from build123d import *

# Parameters (mm, degrees)
F0_W          = 19
F0_H          = 16
F1_DEPTH      = 200
F1_DEPTH_BACK = 25
F3_DEPTH      = 8


with BuildPart() as f1:
    # F0 (on Top) → F1 (new body, two sides)
    with BuildSketch(Plane.XY) as f1_sk:
        with Locations((4.5, 0)):
            Rectangle(F0_W, F0_H)
    extrude(amount=F1_DEPTH)
    extrude(f1_sk.sketch, amount=-F1_DEPTH_BACK)

    # F2 (on Front) → F3 (join, symmetric)
    with BuildSketch(Plane.XZ):
        with BuildLine():
            Line((-7.933333, 193.6), (-5, 191.4))
            Line((-5, 191.4), (-5, 197.4))
            Line((-5, 197.4), (-7.933333, 195.2))
            ThreePointArc((-7.933333, 195.2), (-8.333333, 194.4), (-7.933333, 193.6))
        make_face()
        with BuildLine():
            Line((-7.933333, 185.5), (-5, 183.3))
            Line((-5, 183.3), (-5, 189.3))
            Line((-5, 189.3), (-7.933333, 187.1))
            ThreePointArc((-7.933333, 187.1), (-8.333333, 186.3), (-7.933333, 185.5))
        make_face()
        with BuildLine():
            Line((-7.933333, 177.4), (-5, 175.2))
            Line((-5, 175.2), (-5, 181.2))
            Line((-5, 181.2), (-7.933333, 179))
            ThreePointArc((-7.933333, 179), (-8.333333, 178.2), (-7.933333, 177.4))
        make_face()
        with BuildLine():
            Line((-7.933333, 169.3), (-5, 167.1))
            Line((-5, 167.1), (-5, 173.1))
            Line((-5, 173.1), (-7.933333, 170.9))
            ThreePointArc((-7.933333, 170.9), (-8.333333, 170.1), (-7.933333, 169.3))
        make_face()
        with BuildLine():
            Line((-7.933333, 161.2), (-5, 159))
            Line((-5, 159), (-5, 165))
            Line((-5, 165), (-7.933333, 162.8))
            ThreePointArc((-7.933333, 162.8), (-8.333333, 162), (-7.933333, 161.2))
        make_face()
        with BuildLine():
            Line((-7.933333, 153.1), (-5, 150.9))
            Line((-5, 150.9), (-5, 156.9))
            Line((-5, 156.9), (-7.933333, 154.7))
            ThreePointArc((-7.933333, 154.7), (-8.333333, 153.9), (-7.933333, 153.1))
        make_face()
        with BuildLine():
            Line((-7.933333, 145), (-5, 142.8))
            Line((-5, 142.8), (-5, 148.8))
            Line((-5, 148.8), (-7.933333, 146.6))
            ThreePointArc((-7.933333, 146.6), (-8.333333, 145.8), (-7.933333, 145))
        make_face()
        with BuildLine():
            Line((-7.933333, 136.9), (-5, 134.7))
            Line((-5, 134.7), (-5, 140.7))
            Line((-5, 140.7), (-7.933333, 138.5))
            ThreePointArc((-7.933333, 138.5), (-8.333333, 137.7), (-7.933333, 136.9))
        make_face()
        with BuildLine():
            Line((-7.933333, 128.8), (-5, 126.6))
            Line((-5, 126.6), (-5, 132.6))
            Line((-5, 132.6), (-7.933333, 130.4))
            ThreePointArc((-7.933333, 130.4), (-8.333333, 129.6), (-7.933333, 128.8))
        make_face()
        with BuildLine():
            Line((-7.933333, 120.7), (-5, 118.5))
            Line((-5, 118.5), (-5, 124.5))
            Line((-5, 124.5), (-7.933333, 122.3))
            ThreePointArc((-7.933333, 122.3), (-8.333333, 121.5), (-7.933333, 120.7))
        make_face()
        with BuildLine():
            Line((-7.933333, 112.6), (-5, 110.4))
            Line((-5, 110.4), (-5, 116.4))
            Line((-5, 116.4), (-7.933333, 114.2))
            ThreePointArc((-7.933333, 114.2), (-8.333333, 113.4), (-7.933333, 112.6))
        make_face()
        with BuildLine():
            Line((-7.933333, 104.5), (-5, 102.3))
            Line((-5, 102.3), (-5, 108.3))
            Line((-5, 108.3), (-7.933333, 106.1))
            ThreePointArc((-7.933333, 106.1), (-8.333333, 105.3), (-7.933333, 104.5))
        make_face()
        with BuildLine():
            Line((-7.933333, 96.4), (-5, 94.2))
            Line((-5, 94.2), (-5, 100.2))
            Line((-5, 100.2), (-7.933333, 98))
            ThreePointArc((-7.933333, 98), (-8.333333, 97.2), (-7.933333, 96.4))
        make_face()
        with BuildLine():
            Line((-7.933333, 88.3), (-5, 86.1))
            Line((-5, 86.1), (-5, 92.1))
            Line((-5, 92.1), (-7.933333, 89.9))
            ThreePointArc((-7.933333, 89.9), (-8.333333, 89.1), (-7.933333, 88.3))
        make_face()
        with BuildLine():
            Line((-7.933333, 80.2), (-5, 78))
            Line((-5, 78), (-5, 84))
            Line((-5, 84), (-7.933333, 81.8))
            ThreePointArc((-7.933333, 81.8), (-8.333333, 81), (-7.933333, 80.2))
        make_face()
        with BuildLine():
            Line((-7.933333, 72.1), (-5, 69.9))
            Line((-5, 69.9), (-5, 75.9))
            Line((-5, 75.9), (-7.933333, 73.7))
            ThreePointArc((-7.933333, 73.7), (-8.333333, 72.9), (-7.933333, 72.1))
        make_face()
        with BuildLine():
            Line((-7.933333, 64), (-5, 61.8))
            Line((-5, 61.8), (-5, 67.8))
            Line((-5, 67.8), (-7.933333, 65.6))
            ThreePointArc((-7.933333, 65.6), (-8.333333, 64.8), (-7.933333, 64))
        make_face()
        with BuildLine():
            Line((-7.933333, 55.9), (-5, 53.7))
            Line((-5, 53.7), (-5, 59.7))
            Line((-5, 59.7), (-7.933333, 57.5))
            ThreePointArc((-7.933333, 57.5), (-8.333333, 56.7), (-7.933333, 55.9))
        make_face()
        with BuildLine():
            Line((-7.933333, 47.8), (-5, 45.6))
            Line((-5, 45.6), (-5, 51.6))
            Line((-5, 51.6), (-7.933333, 49.4))
            ThreePointArc((-7.933333, 49.4), (-8.333333, 48.6), (-7.933333, 47.8))
        make_face()
        with BuildLine():
            Line((-7.933333, 39.7), (-5, 37.5))
            Line((-5, 37.5), (-5, 43.5))
            Line((-5, 43.5), (-7.933333, 41.3))
            ThreePointArc((-7.933333, 41.3), (-8.333333, 40.5), (-7.933333, 39.7))
        make_face()
        with BuildLine():
            Line((-7.933333, 31.6), (-5, 29.4))
            Line((-5, 29.4), (-5, 35.4))
            Line((-5, 35.4), (-7.933333, 33.2))
            ThreePointArc((-7.933333, 33.2), (-8.333333, 32.4), (-7.933333, 31.6))
        make_face()
        with BuildLine():
            Line((-7.933333, 23.5), (-5, 21.3))
            Line((-5, 21.3), (-5, 27.3))
            Line((-5, 27.3), (-7.933333, 25.1))
            ThreePointArc((-7.933333, 25.1), (-8.333333, 24.3), (-7.933333, 23.5))
        make_face()
        with BuildLine():
            Line((-7.933333, 15.4), (-5, 13.2))
            Line((-5, 13.2), (-5, 19.2))
            Line((-5, 19.2), (-7.933333, 17))
            ThreePointArc((-7.933333, 17), (-8.333333, 16.2), (-7.933333, 15.4))
        make_face()
        with BuildLine():
            Line((-7.933333, 7.3), (-5, 5.1))
            Line((-5, 5.1), (-5, 11.1))
            Line((-5, 11.1), (-7.933333, 8.9))
            ThreePointArc((-7.933333, 8.9), (-8.333333, 8.1), (-7.933333, 7.3))
        make_face()
        with BuildLine():
            Line((-5, 3), (-7.933333, 0.8))
            ThreePointArc((-7.933333, 0.8), (-8.333333, 0), (-7.933333, -0.8))
            Line((-7.933333, -0.8), (-5, -3))
            Line((-5, -3), (-5, 3))
        make_face()
    extrude(amount=F3_DEPTH, both=True)


solid = f1.part
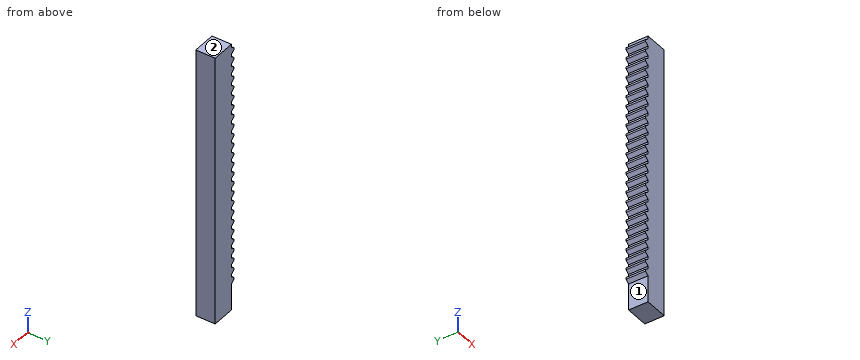
The listing builds one solid part. Answer for the finished solid, in the listing's coordinates (mm). Face numbers are marked on the shaded views. A direction names the side the tool comes from. Give positions to 0.01 mm unless a question says otherwise; leave off trailing zeros. Use a Markdown table: item, result.
1. A tool of negligible diameter and unlimited length cuts with its end or side. For the marked faces 1 and 2, from which of +Z, -Z, +X, -X, +Y, -Y can it reach the whole face along a straight path? Write none if from no direction.
Values follow:
| item | result |
|---|---|
| face 1 | -Z, -X, +Y, -Y |
| face 2 | +Z, +X, -X, +Y, -Y |
2. Find the intervals of material crossed by probe 1 along X at (y, z) = (2.75, 133); probe 2 along X at (y, z) = (-3.25, 73), in increasing order. Write a range as from..to.
Values follow:
| item | result |
|---|---|
| probe 1 | x = -5..14 |
| probe 2 | x = -8.33..14 |
3. Each of these flat-tipped pins is pushed along its axis until it touches: P1, Ø1.7, axis at y = 2, z = 69, coming from the -X side; P2, Ø2.5, axis at y = -1, z = 149.5, coming from the -X side; P3, Ø2.5, axis at y = 2, z = 125, coming from the -X side. Where does it stop, or does it pass through?
Values follow:
| item | result |
|---|---|
| P1 | stops at x = -5 |
| P2 | stops at x = -5.73 |
| P3 | stops at x = -6 |
